Autodesk Inventor part; units mm, degrees
ref_plane "YZ Plane" through (0, 0, 0) normal (1, 0, 0) x (0, 1, 0)
ref_plane "XZ Plane" through (0, 0, 0) normal (0, 1, 0) x (-1, 0, 0)
ref_plane "XY Plane" through (0, 0, 0) normal (0, 0, 1) x (1, 0, 0)
sketch "Sketch1" plane through (0, 0, 0) normal (0, 0, 1) x (1, 0, 0)
  line L0 (0, 21.5799) -> (0, -21.5799)
  line L1 (-172.0799, 0) -> (172.0799, 0)
  line L2 (-120.5, 15) -> (120.5, 15)
  line L3 (122.5, 13) -> (122.5, -13)
  line L4 (-122.5, -13) -> (-122.5, 13)
  arc A0 (-21.6071, 2.3273) -> (-28.3929, 2.3273) centre (-25, 6) ccw
  line L5 (-25, 6) -> (-25, -2.9295)
  line L6 (-27.75, 0.8583) -> (-27.75, -13)
  line L7 (-22.25, 0.8583) -> (-22.25, -13)
  arc A1 (-27.75, 0.8583) -> (-28.3929, 2.3273) centre (-29.75, 0.8583) ccw
  arc A2 (-21.6071, 2.3273) -> (-22.25, 0.8583) centre (-20.25, 0.8583) ccw
  arc A3 (-29.75, -15) -> (-27.75, -13) centre (-29.75, -13) ccw
  arc A4 (-22.25, -13) -> (-20.25, -15) centre (-20.25, -13) ccw
  arc A5 (-71.6071, 2.3273) -> (-78.3929, 2.3273) centre (-75, 6) ccw
  line L8 (-75, 6) -> (-75, -2.9295)
  line L9 (-77.75, 0.8583) -> (-77.75, -13)
  line L10 (-72.25, 0.8583) -> (-72.25, -13)
  arc A6 (-77.75, 0.8583) -> (-78.3929, 2.3273) centre (-79.75, 0.8583) ccw
  arc A7 (-71.6071, 2.3273) -> (-72.25, 0.8583) centre (-70.25, 0.8583) ccw
  arc A8 (-79.75, -15) -> (-77.75, -13) centre (-79.75, -13) ccw
  arc A9 (-72.25, -13) -> (-70.25, -15) centre (-70.25, -13) ccw
  line L11 (-29.75, -15) -> (-70.25, -15)
  line L12 (-79.75, -15) -> (-120.5, -15)
  arc A10 (28.3929, 2.3273) -> (21.6071, 2.3273) centre (25, 6) ccw
  line L13 (25, 6) -> (25, -2.9295)
  line L14 (27.75, 0.8583) -> (27.75, -13)
  line L15 (22.25, 0.8583) -> (22.25, -13)
  arc A11 (28.3929, 2.3273) -> (27.75, 0.8583) centre (29.75, 0.8583) ccw
  arc A12 (22.25, 0.8583) -> (21.6071, 2.3273) centre (20.25, 0.8583) ccw
  arc A13 (27.75, -13) -> (29.75, -15) centre (29.75, -13) ccw
  arc A14 (20.25, -15) -> (22.25, -13) centre (20.25, -13) ccw
  line L16 (72.25, 0.8583) -> (72.25, -13)
  arc A15 (72.25, 0.8583) -> (71.6071, 2.3273) centre (70.25, 0.8583) ccw
  arc A16 (70.25, -15) -> (72.25, -13) centre (70.25, -13) ccw
  arc A17 (78.3929, 2.3273) -> (71.6071, 2.3273) centre (75, 6) ccw
  line L17 (77.75, 0.8583) -> (77.75, -13)
  arc A18 (78.3929, 2.3273) -> (77.75, 0.8583) centre (79.75, 0.8583) ccw
  line L18 (75, 6) -> (75, -2.9295)
  arc A19 (77.75, -13) -> (79.75, -15) centre (79.75, -13) ccw
  line L19 (20.25, -15) -> (-20.25, -15)
  line L20 (120.5, -15) -> (79.75, -15)
  line L21 (70.25, -15) -> (29.75, -15)
  arc A20 (-120.5, 15) -> (-122.5, 13) centre (-120.5, 13) ccw
  arc A21 (-122.5, -13) -> (-120.5, -15) centre (-120.5, -13) ccw
  arc A22 (120.5, -15) -> (122.5, -13) centre (120.5, -13) ccw
  arc A23 (122.5, 13) -> (120.5, 15) centre (120.5, 13) ccw
  point P0 (0, 0)
  point P1 (-122.5, 15)
  point P2 (122.5, 15)
  point P3 (-122.5, -15)
  point P4 (-27.75, 1.8242)
  point P5 (-22.25, 1.8242)
  point P6 (-77.75, 1.8242)
  point P7 (-72.25, 1.8242)
  point P8 (27.75, 1.8242)
  point P9 (22.25, 1.8242)
  point P10 (72.25, 1.8242)
  point P11 (77.75, 1.8242)
  dimension "d0" = 245
  dimension "d1" = 30
  dimension "d2" = 10
  dimension "d3" = 25
  dimension "d4" = 6
  dimension "d5" = 5.5
  dimension "d6" = 2
  dimension "d7" = 2
  dimension "d9" = 10
  dimension "d10" = 5.5
  dimension "d11" = 2
  dimension "d12" = 2
  dimension "d13" = 2
  dimension "d14" = 50
extrude "Extrusion1" add sketch "Sketch1" against normal blind 15 contours L2 A23 L3 L1 L17 A18 A17 A15 L16 L14 A11 A10 A12 L15 L0 | L0 L1 L7 A2 A0 A1 L6 L10 A7 A5 A6 L9 L4 A20 L2 | L1 L15 A14 L19 L0 | L0 L19 A4 L7 L1 | L1 L9 A8 L12 A21 L4 | L3 A22 L20 A19 L17 L1 | L6 A3 L11 A9 L10 L1 | L1 L16 A16 L21 A13 L14
properties part number "SlipersLåda 211018007"
The model under review builds one solid part; all positions refer to its coordinate system, in mm. A direction names the side the tool comes from. Coordinates: 2 decimals unless noted, no trailing zeros. Write each loop counter-clockwise with the first axis right and the second up, starting at its lowest first coordinate (ties: lowest second). Pieces come first, ordered by that corner, then holes. Notation, with made-up numbers: (-3.5, -12.75) - (7.5, -12.75) arc R22 cw to (7.5, 3.25) - close; hole circle Ø3 at (-30, 12.5). An arc over 180 degrees is marked (long way). Answer as CSV lines item,"result".
(1) We need section A-A (y = 6). Give the boundary of the cut face in (x, z), plus the area to 4 significant figures.
Data:
outline,"(-122.5, -15) - (-80, -15) - (-80, 0) - (-122.5, 0) - close; (-70, -15) - (-30, -15) - (-30, 0) - (-70, 0) - close; (-20, -15) - (20, -15) - (20, 0) - (-20, 0) - close; (30, -15) - (70, -15) - (70, 0) - (30, 0) - close; (80, -15) - (122.5, -15) - (122.5, 0) - (80, 0) - close"
area,"3,075 mm2"
(2) Clearance check with a flat-ended pin moving along its axis: pin 1 Ø9 at (x, y) = (75, 6) entering from +Z. State where the tip first meets the part, or that it passes through.
Data:
pin 1,"passes through"
(3) Tool access review of faces 1 (the flat face through (72.25, -6, -7)), 2 (the cylindrical face through (75, 11, -7)): name each direction out of +Z, -Z, +X, -X, +Y, -Y from which nothing blocks a thin tool from reaching the whole face with its end or side.
Data:
face 1,"+Z, -Z, -Y"
face 2,"+Z, -Z"
(4) We need section B-B (y = -3.75). Give the boundary of the cut face in (x, z).
Data:
outline,"(-122.5, -15) - (-77.75, -15) - (-77.75, 0) - (-122.5, 0) - close; (-72.25, -15) - (-27.75, -15) - (-27.75, 0) - (-72.25, 0) - close; (-22.25, -15) - (22.25, -15) - (22.25, 0) - (-22.25, 0) - close; (27.75, -15) - (72.25, -15) - (72.25, 0) - (27.75, 0) - close; (77.75, -15) - (122.5, -15) - (122.5, 0) - (77.75, 0) - close"
(5) Mouldability with a two-part tool opening along X and no side actions: class faces 3 (the flat face through (-77.75, -6, -7)), 4 (the flat face through (-122.5, 0, -7)), 5 (the flat face through (122.5, 0, -7)), 6 (the flat face through (50, -15, -7)) as pulls with the +X half, pulls with the -X half, needs draft (parallel to the pull), parting line crosses it, or undercut.
Data:
face 3,"undercut"
face 4,"pulls with the -X half"
face 5,"pulls with the +X half"
face 6,"needs draft"
(6) For line 1 along X through (y, z) = (6, -8); line 2 along X through (y, z) = (-6.5, -4.5); line 3 along Y through (x, z) = (-75, -6.25), list the stretches that pass through material, from the lowest coordinate up. Write a range as [from, to].
Data:
line 1,"x = [-122.5, -80], [-70, -30], [-20, 20], [30, 70], [80, 122.5]"
line 2,"x = [-122.5, -77.75], [-72.25, -27.75], [-22.25, 22.25], [27.75, 72.25], [77.75, 122.5]"
line 3,"y = [11, 15]"
(7) We need section C-C (x = -25). Give the boundary of the cut face in (y, z).
Data:
outline,"(11, -15) - (15, -15) - (15, 0) - (11, 0) - close"
